from build123d import *

# Parameters (mm, degrees)
F1_DEPTH = 63.5
F3_DEPTH = 127
F5_D     = 12.7


with BuildPart() as f1:
    # F0 (on Top) → F1 (new body)
    with BuildSketch(Plane.XY):
        Polygon((-35.944343, 50.081447), (-35.944343, 0), (-35.944343, -50.081447), (0, -50.081447), (35.944343, -50.081447), (35.944343, 0), (35.944343, 50.081447), (0, 50.081447), align=None)
        Polygon((-28.725395, -42.862501), (-28.725395, 0), (-28.725395, 42.862501), (0, 42.862501), (28.725395, 42.862501), (28.725395, 0), (28.725395, -42.862501), (0, -42.862501), align=None, mode=Mode.SUBTRACT)
    extrude(amount=F1_DEPTH)

    # F2 (on face) → F3 (cut)
    with BuildSketch(Plane.YZ.offset(35.944343)):
        Polygon((20.60408, 63.5), (-20.60408, 63.5), (-20.60408, 40.456183), (0, 40.456183), (20.60408, 40.456183), align=None)
    extrude(amount=-F3_DEPTH, mode=Mode.SUBTRACT)

    # F5 (through all)
    with Locations(Plane.XZ.offset(50.081447)):
        with Locations((0, 47.073554)):
            Hole(F5_D / 2)


solid = f1.part
Model file for the job. Use its own axes, mm. A direction names the side the tool comes from. Round coordinates to 2 decimals unless told otherwise and drop trailing zeros. Loops run counter-clockwise (first coordinate to the right, second up) from the corner with the lowest first, then second, coordinate; pieces in that order, holes last.
1. Band-saw the part on D-D, the plane x = 0. List the corners of the cut face in (y, z).
Check values:
outline: (-50.08, 0) - (-42.86, 0) - (-42.86, 40.72) - (-50.08, 40.72) - close; (-50.08, 53.42) - (-42.86, 53.42) - (-42.86, 63.5) - (-50.08, 63.5) - close; (42.86, 0) - (50.08, 0) - (50.08, 40.72) - (42.86, 40.72) - close; (42.86, 53.42) - (50.08, 53.42) - (50.08, 63.5) - (42.86, 63.5) - close
2. Band-saw the part on C-C, the plane x = -18. List the corners of the cut face in (y, z), and give its area (3 significant figures).
Check values:
outline: (-50.08, 0) - (-42.86, 0) - (-42.86, 63.5) - (-50.08, 63.5) - close; (42.86, 0) - (50.08, 0) - (50.08, 63.5) - (42.86, 63.5) - close
area: 917 mm2
3. Drop flat-ended pins along their axis: P1, Ø10, axis at x = 0, z = 47.07, coming from the -Y side; P2, Ø6, axis at x = -31.5, y = -5, coming from the +Z side. Give the stop position or say it passes through.
Check values:
P1: passes through
P2: stops at z = 40.46
4. Tool access for faces 5 (the flat face through (-28.725, -1, 24)), 6 (the flat face through (32, 20.604, 52)), 7 (the flat face through (-1, -45, 63.5)): list every direction of +Z, -Z, +X, -X, +Y, -Y with a clear straight run to the whole face (end or side of a thin tool).
Check values:
face 5: +Z, -Z
face 6: +Z, +X, -X
face 7: +Z, +X, -X, +Y, -Y
5. Band-saw the part on A-A, the plane z = 56. List the corners of the cut face in (x, y), and give its area (3 significant figures).
Check values:
outline: (-35.94, -50.08) - (35.94, -50.08) - (35.94, -20.6) - (28.73, -20.6) - (28.73, -42.86) - (-28.73, -42.86) - (-28.73, -20.6) - (-35.94, -20.6) - close; (-35.94, 20.6) - (-28.73, 20.6) - (-28.73, 42.86) - (28.73, 42.86) - (28.73, 20.6) - (35.94, 20.6) - (35.94, 50.08) - (-35.94, 50.08) - close
area: 1,680 mm2
6. Band-saw the part on B-B, the plane y = 10. List the corners of the cut face in (x, z), and give its area (3 significant figures).
Check values:
outline: (-35.94, 0) - (-28.73, 0) - (-28.73, 40.46) - (-35.94, 40.46) - close; (28.73, 0) - (35.94, 0) - (35.94, 40.46) - (28.73, 40.46) - close
area: 584 mm2
7. Wall check: probe 1 along Z at (x, y) = (0, 46); probe 2 along X at (y, z) = (37, 50.5); probe 3 along Y at (x, z) = (28, 23.5). Give the ranges that are in metal, low to high.
Check values:
probe 1: z = 0 to 40.72, 53.42 to 63.5
probe 2: x = -35.94 to -28.73, 28.73 to 35.94
probe 3: y = -50.08 to -42.86, 42.86 to 50.08
8. Mould opens along X. For faces 1 (the flat face through (28.725, 1, 24)), 2 (the flat face through (0, 42.863, 31)), 3 (the flat face through (-32, -20.604, 52)), 4 (the flat face through (35.944, -1, 31)) say: +X half, -X half, draft (parallel to the pull), parting line (faces both ways), or undercut.
Check values:
face 1: undercut
face 2: undercut
face 3: draft
face 4: +X half
